CAD build for the part. Positions are in the model's coordinates, mm. A direction names the side the tool comes from. Coordinates: 2 decimals unless noted, no trailing zeros. Write each loop counter-clockwise with the first axis right and the second up, starting at its lowest first coordinate (ties: lowest second). Pieces come first, ordered by that corner, then holes.
```python
from build123d import *

# Parameters (mm, degrees)
SKETCH_W   = 40
SKETCH_H   = 68
SKETCH_R   = 1.5
SKETCH_W_2 = 23
SKETCH_H_2 = 2.5
PAD_DEPTH  = 0.825


with BuildPart() as part:
    # Sketch → Pad (new body, symmetric)
    with BuildSketch(Plane.XY):
        Rectangle(SKETCH_W, SKETCH_H)
        with Locations((-17.1, 31.25)):
            Circle(SKETCH_R, mode=Mode.SUBTRACT)
        with Locations((17.1, 31.25)):
            Circle(SKETCH_R, mode=Mode.SUBTRACT)
        with Locations((-17.1, -31.25)):
            Circle(SKETCH_R, mode=Mode.SUBTRACT)
        with Locations((17.1, -31.25)):
            Circle(SKETCH_R, mode=Mode.SUBTRACT)
        with Locations((0, 32.25)):
            Rectangle(SKETCH_W_2, SKETCH_H_2, mode=Mode.SUBTRACT)
    extrude(amount=PAD_DEPTH, both=True)


solid = part.part
```
Item 1: Saw through at C-C, the plane x = -7.5. Write the cut outline in (y, z) (3 decimals).
Item 2: Two-plate mould, pull along Y, no slides. Class faces 1 (the flat face through (0, -34, 0)), 2 (the flat face through (11.5, 32, 0)), 3 (the flat face through (0, 31, 0)), 4 (the flat face through (-20, 0, 0)): +Y half, -Y half, draft (parallel to the pull), parting line (faces both ways), or undercut.
Item 3: Saw through at A-A, the plane x = 17.1. Write the cut outline in (y, z) (3 decimals).
Item 4: Which spindle directions (+Z, -Z, +X, -X, +Y, -Y) get a long thin tool onto all of the face, cutting with end or side? Do faces 5 (the flat face through (-11.5, 32, 0)), 6 (the flat face through (0, 0, 0.825)). Say none if no direction does.
Item 5: Wall check: line 1 along Y through (x, z) = (17.1, -0.35); line 2 along Y through (x, z) = (-8, 0.2); line 3 along Y through (x, z) = (18, 0.2). Give the ranges that are in metal, low to high.
Item 6: Flat gauge pins, fed straight in: pin 1 Ø1.8 at (x, y) = (17.1, -31.25) entering from -Z; pin 2 Ø4 at (x, y) = (17.1, 31.25) entering from -Z (3 decimals). Where does each tip first touch, or does it go through?
Item 7: Saw through at B-B, the plane z = 0.05. Write the cut outline in (x, y).
Item 8: Saw through at D-D, the plane y = -31.25. Write the cut outline in (x, z) (3 decimals), and give its area (3 significant figures).
Working result:
1. outline: (-34, -0.825) - (31, -0.825) - (31, 0.825) - (-34, 0.825) - close; (33.5, -0.825) - (34, -0.825) - (34, 0.825) - (33.5, 0.825) - close
2. face 1: -Y half
2. face 2: undercut
2. face 3: undercut
2. face 4: draft
3. outline: (-34, -0.825) - (-32.75, -0.825) - (-32.75, 0.825) - (-34, 0.825) - close; (-29.75, -0.825) - (29.75, -0.825) - (29.75, 0.825) - (-29.75, 0.825) - close; (32.75, -0.825) - (34, -0.825) - (34, 0.825) - (32.75, 0.825) - close
4. face 5: +Z, -Z
4. face 6: +Z, +X, -X, +Y, -Y
5. line 1: y = -34 to -32.75, -29.75 to 29.75, 32.75 to 34
5. line 2: y = -34 to 31, 33.5 to 34
5. line 3: y = -34 to -32.45, -30.05 to 30.05, 32.45 to 34
6. pin 1: passes through
6. pin 2: stops at z = -0.825
7. outline: (-20, -34) - (20, -34) - (20, 34) - (-20, 34) - close; hole circle Ø3 at (-17.1, -31.25); hole circle Ø3 at (-17.1, 31.25); hole (-11.5, 31) - (11.5, 31) - (11.5, 33.5) - (-11.5, 33.5) - close; hole circle Ø3 at (17.1, -31.25); hole circle Ø3 at (17.1, 31.25)
8. outline: (-20, -0.825) - (-18.6, -0.825) - (-18.6, 0.825) - (-20, 0.825) - close; (-15.6, -0.825) - (15.6, -0.825) - (15.6, 0.825) - (-15.6, 0.825) - close; (18.6, -0.825) - (20, -0.825) - (20, 0.825) - (18.6, 0.825) - close
8. area: 56.1 mm2
